The drawing under review shows one solid part. Ordinate dimensions are in mm from its lowest x, y, z. A direction names the side the tool comes from. Round coordinates to 2 decimals unless told otherwise and drop trailing zeros. Order: outer loops, then holes, each group sorted by start corner. A loop starts at its lowest first (then second) coordinate and runs counter-clockwise, first axis right, second up. Notation, with made-up numbers: M -3.75,20 L 35.25,20 A25 cw 35.25,44 Z; hole C 47,79.5 d5. An arc over 180 degrees is marked long. Answer as a JSON object with one key per item and string values.
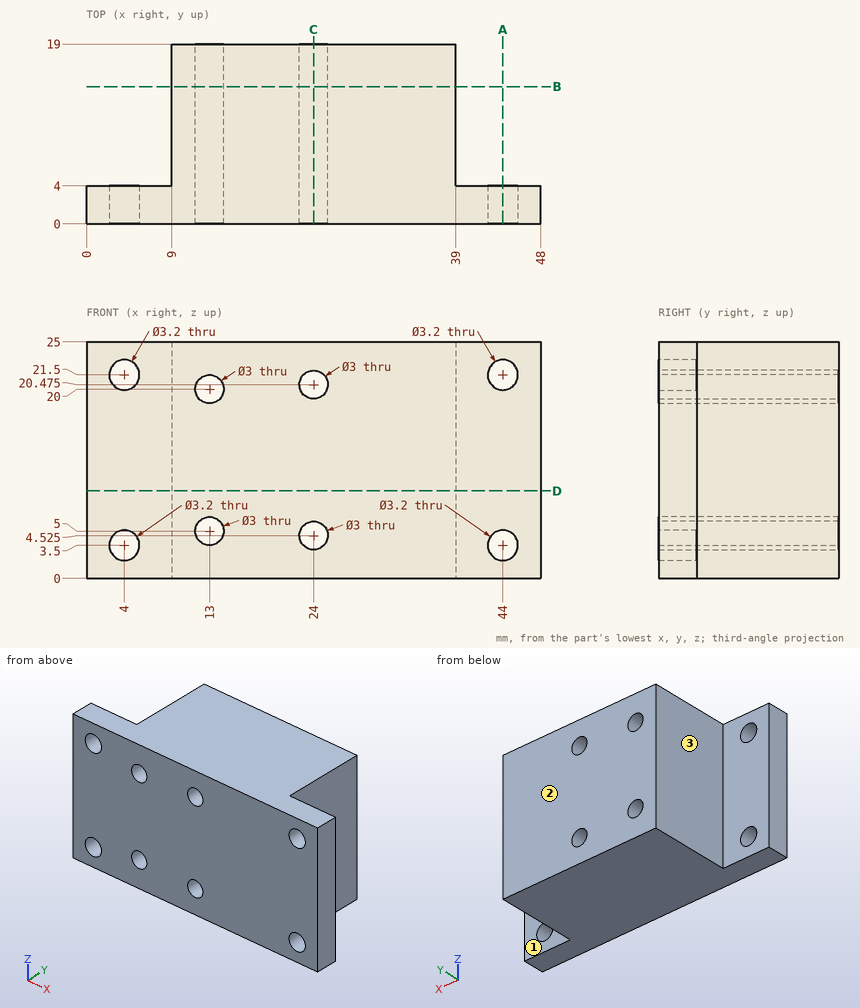
1) Add section A-A on x = 44. State the section outline as (y, z) points.
Geometry check:
{"outline": "M 0,0 L 4,0 L 4,1.9 L 0,1.9 Z; M 0,5.1 L 4,5.1 L 4,19.9 L 0,19.9 Z; M 0,23.1 L 4,23.1 L 4,25 L 0,25 Z"}
2) Add section C-C on x = 24. State the section outline as (y, z) points (3 decimals).
Geometry check:
{"outline": "M 0,0 L 19,0 L 19,3.025 L 0,3.025 Z; M 0,6.025 L 19,6.025 L 19,18.975 L 0,18.975 Z; M 0,21.975 L 19,21.975 L 19,25 L 0,25 Z"}
3) Add section D-D on z = 9.25. State the section outline as (x, y) points.
Geometry check:
{"outline": "M 0,0 L 48,0 L 48,4 L 39,4 L 39,19 L 9,19 L 9,4 L 0,4 Z"}
4) Insertion check: P1, Ø3.5, axis at x = 44, z = 21.5, coming from the +Y side; P2, Ø1.5, axis at y = 8.5, z = 4.5, coming from the -X side; P3, Ø12, axis at x = 33.5, z = 15, coming from the -Y side; P4, Ø1.8, axis at x = 13, z = 5, coming from the -Y side. Each pin has a flat end and moves straight along its axis. Give the tip position at first contact, or say it passes through.
Geometry check:
{"P1": "stops at y = 4", "P2": "stops at x = 9", "P3": "stops at y = 0", "P4": "passes through"}
5) For L1, parallel to X at y = 9.5, z = 20; L2, parallel to X at y = 17, z = 22.75; L3, parallel to X at y = 14.5, z = 5.5, list the stretches that pass through material, from the lowest coordinate up.
Geometry check:
{"L1": "x = 9 to 11.5, 14.5 to 22.58, 25.42 to 39", "L2": "x = 9 to 39", "L3": "x = 9 to 11.59, 14.41 to 22.86, 25.14 to 39"}
6) Add section B-B on y = 14.5. State the section outline as (x, z) points (3 decimals).
Geometry check:
{"outline": "M 9,0 L 39,0 L 39,25 L 9,25 Z; hole C 13,5 d3; hole C 13,20 d3; hole C 24,4.525 d3; hole C 24,20.475 d3"}
7) Machinability: for the marked faces 1, 2 and 3, which of the approach directions +Z, -Z, +X, -X, +Y, -Y give a long, thin tool a straight path to every point of the face, cutting with its end or side? Answer none if there is none.
Geometry check:
{"face 1": "+Z, -Z, +X, +Y", "face 2": "+Z, -Z, +X, -X, +Y", "face 3": "+Z, -Z, -X, +Y"}
